Read the model definition and answer for the solid it produces. Units are mm, in the model's axes. A direction names the side the tool comes from. Give positions to 0.01 mm unless a question says otherwise; leave off trailing zeros. Loops run counter-clockwise (first coordinate to the right, second up) from the corner with the lowest first, then second, coordinate; pieces in that order, holes last. Notation, with made-up numbers: M -37,29 L -8,29 A24 ccw -8,48 Z; hole C 51,14.5 d3. An arc over 180 degrees is marked long. Return JSON: item names as keys, results as strings. Group by question number.
Autodesk Fusion 360 part; units mm, degrees
sketch "Sketch3" plane through (0, 0, 0) normal (0, 1, 0) x (1, 0, 0)
sketch "Sketch4" plane through (0, 0, 0) normal (0, 1, 0) x (1, 0, 0)
sketch "Sketch5" plane through (0, 0, 0) normal (0, 1, 0) x (1, 0, 0)
sketch "Sketch6" plane through (0, 0, 0) normal (0, 1, 0) x (1, 0, 0)
  line L0 (-42.6895, -21.6471) -> (19.3705, -21.6471)
  line L1 (19.3705, -21.6471) -> (19.3705, 29.8529)
  line L2 (19.3705, 29.8529) -> (-42.6895, 29.8529)
  line L3 (-42.6895, 29.8529) -> (-42.6895, -21.6471)
  line L4 (-52.6895, -31.6471) -> (29.3705, -31.6471)
  line L5 (29.3705, -31.6471) -> (29.3705, 39.8529)
  line L6 (29.3705, 39.8529) -> (-52.6895, 39.8529)
  line L7 (-52.6895, 39.8529) -> (-52.6895, -31.6471)
  circle A0 centre (-47.6895, -26.6471) radius 1.45
  circle A1 centre (24.3705, -26.6471) radius 1.45
  circle A2 centre (-47.6895, 34.8529) radius 1.45
  circle A3 centre (24.3705, 34.8529) radius 1.45
  dimension "d52" = 51.5
  dimension "d53" = 62.06
  dimension "d54" = 10
  dimension "d55" = 10
  dimension "d56" = 10
  dimension "d57" = 10
  dimension "d58" = 2.9
  dimension "d59" = 5
  dimension "d60" = 5
  dimension "d61" = 2.9
  dimension "d62" = 5
  dimension "d63" = 5
  dimension "d64" = 2.9
  dimension "d65" = 5
  dimension "d66" = 5
  dimension "d67" = 2.9
  dimension "d68" = 5
  dimension "d69" = 5
extrude "Extrude6" add sketch "Sketch6" along normal blind 13
extrude "Extrude7" add sketch "Sketch6" along normal blind 3 contours L0 L1 L2 L3
sketch "Sketch7" plane through (0, 0, 0) normal (0, 1, 0) x (1, 0, 0)
  line L0 (13.2505, -31.6778) -> (4.2505, -31.6778)
  line L1 (4.2505, -31.6778) -> (4.2505, -21.6778)
  line L2 (4.2505, -21.6778) -> (13.2505, -21.6778)
  line L3 (13.2505, -21.6778) -> (13.2505, -31.6778)
  line L4 (19.3705, -21.6471) -> (19.3705, 29.8529)
  dimension "d74" = 10
  dimension "d75" = 6.12
  dimension "d76" = 9
sketch "Sketch8" plane through (0, 0, 0) normal (0, 1, 0) x (1, 0, 0)
sketch "eee" plane through (0, 0, 0) normal (0, 1, 0) x (1, 0, 0)
  line L0 (13.3073, -31.6778) -> (4.2109, -31.6778)
  line L1 (4.2109, -31.6778) -> (4.2109, -21.6873)
  line L2 (4.2109, -21.6873) -> (13.3073, -21.6873)
  line L3 (13.3073, -21.6873) -> (13.3073, -31.6778)
  line L4 (4.2505, -21.6778) -> (13.2505, -21.6778)
  dimension "d77" = 10
extrude "Extrude8" cut sketch "eee" along normal blind 13
1. A flat-ended cylindrical pin translates along its axis: P1, Ø2.5, axis at x = 9, y = 8, coming from the +Z side. Find the tip coordinate at first contact, or state that the pin passes through.
2. For faces 1 (the flat face through (13.307, 6, 27)), 2 (the flat face through (-42.69, 8, -4)), 3 (the cylindrical face through (25.71, 6.41, 26.09)), determine the directions among +Z, -Z, +X, -X, +Y, -Y from which every point of the face is accessible in a straight line to the end or side of a thin tool.
3. The mould has two halves that part along X. Classify faces 4 (the flat face through (-11, 8, -29.853)), 5 (the flat face through (-18, 13, -31)), 6 (the flat face through (-52.69, 6, -5)), 7 (the cylindrical face through (-46.91, 6.41, -33.63)): +X half, -X half, draft (parallel to the pull), parting line (faces both ways), or undercut.
4. Find section B-B (z = 11.5). Write down the section's boundary in (x, y).
5. Straight lines are drawn through the part: line 1 along Z through (x, y) = (-6, 8); line 2 along X through (y, z) = (10.5, -23); line 3 along Z through (x, y) = (24, 11.25). For each, find the intervals that lie inside material, in ascending order.
6. Find section C-C (x = -4). Write down the section's boundary in (y, z), and give its area (4 significant figures).
7. Find section A-A (y = 4.5). Write down the section's boundary in (x, z).
Result:
{
 "1": {"P1": "stops at z = 21.69"},
 "2": {"face 1": "+Z, +Y, -Y", "face 2": "+Y", "face 3": "+Y, -Y"},
 "3": {"face 4": "undercut", "face 5": "draft", "face 6": "-X half", "face 7": "undercut"},
 "4": {"outline": "M -52.69,0 L 29.37,0 L 29.37,13 L 19.37,13 L 19.37,3 L -42.69,3 L -42.69,13 L -52.69,13 Z"},
 "5": {"line 1": "z = -39.85 to -29.85, 21.65 to 31.65", "line 2": "x = -52.69 to -42.69, 19.37 to 29.37", "line 3": "z = -39.85 to -36.25, -33.45 to 25.25, 28.05 to 31.65"},
 "6": {"outline": "M 0,-39.85 L 13,-39.85 L 13,-29.85 L 3,-29.85 L 3,21.65 L 13,21.65 L 13,31.65 L 0,31.65 Z", "area": "414.5 mm2"},
 "7": {"outline": "M -52.69,-39.85 L 29.37,-39.85 L 29.37,31.65 L 13.31,31.65 L 13.31,21.69 L 4.21,21.69 L 4.21,31.65 L -52.69,31.65 Z; hole C -47.69,-34.85 d2.9; hole C -47.69,26.65 d2.9; hole M -42.69,-29.85 L 19.37,-29.85 L 19.37,21.65 L -42.69,21.65 Z; hole C 24.37,-34.85 d2.9; hole C 24.37,26.65 d2.9"}
}
